from build123d import *

# Parameters (mm, degrees)
SKETCH1_R           = 25.4
BOSS_EXTRUDE1_DEPTH = 81.407
SKETCH2_R           = 3.81
CUT_EXTRUDE2_DEPTH  = 167.729477286


with BuildPart() as part:
    # Sketch1 → Boss-Extrude1 (new, symmetric)
    with BuildSketch(Plane.XY):
        Circle(SKETCH1_R)
    extrude(amount=BOSS_EXTRUDE1_DEPTH, both=True)

    # Sketch2 → Cut-Extrude2 (cut, through all)
    with BuildSketch(Plane.XY.offset(81.407)):
        Circle(SKETCH2_R)
    extrude(amount=-CUT_EXTRUDE2_DEPTH, mode=Mode.SUBTRACT)

    # Sketch6 → Cut-Revolve1 (revolve, cut)
    with BuildSketch(Plane(origin=(0, 0, 0), x_dir=(0, 0, -1), z_dir=(1, 0, 0)), mode=Mode.PRIVATE) as cut_revolve1_sk:
        Polygon((-12.207313926, 0), (-81.407, 18.542), (-81.407, 0), align=None)
    revolve(cut_revolve1_sk.sketch.rotate(Axis((0, 0, -89.5477), (0, 0, 1)), 270), axis=Axis((0, 0, -89.5477), (0, 0, 1)), mode=Mode.SUBTRACT)


solid = part.part
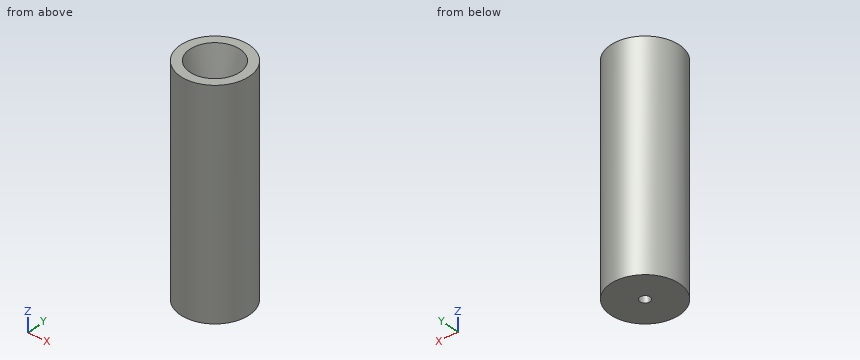
Read the model definition and answer for the solid it produces. Units are mm, in the model's axes. Give positions to 0.01 mm unless a question says otherwise; leave off trailing zeros. Write each loop counter-clockwise with the first axis right and the second up, starting at its lowest first coordinate (ties: lowest second). Pieces come first, ordered by that corner, then holes. Notation, with made-up numbers: (71.5, 52.5) -> (113.5, 52.5) arc R11 ccw to (113.5, 61.5) -> close; hole circle Ø5 at (-8, 0.5). An arc over 180 degrees is marked (long way). Answer as a JSON object with one key per item and string values. Group by question number.
1) Consider L1, parallel to Y at x = 0, z = -32; L2, parallel to Y at x = -3.5, z = -52; L3, parallel to Y at x = -9, z = -16. Determine where each line is inside the solid, lowest interval first. Write a range as from..to.
2) Find section D-D (y = -21.5). Write down the section's boundary in (x, z), and give its area (3 significant figures).
3) Find section C-C (z = -64). Write down the section's boundary in (x, y).
4) Each of these flat-tipped pins is pushed along its axis until it touches: P1, Ø8, axis at x = -10, z = 25.5, coming from the +Y side; P2, Ø2, axis at y = 13, z = 23.5, coming from the -X side; P3, Ø12, axis at y = -12.5, z = -44, coming from the +X side. Where does it stop, or does it pass through?
5) Find section A-A (y = 0). Write down the section's boundary in (x, z), and give its area (3 significant figures).
Values follow:
{
 "1": {"L1": "y = -25.4..-3.81, 3.81..25.4", "L2": "y = -25.16..-1.51, 1.51..25.16", "L3": "y = -23.75..23.75"},
 "2": {"outline": "(-13.52, -81.41) -> (13.52, -81.41) -> (13.52, 81.41) -> (-13.52, 81.41) -> close", "area": "4,400 mm2"},
 "3": {"outline": "circle Ø50.8 at (0, 0); hole circle Ø7.62 at (0, 0)"},
 "4": {"P1": "stops at y = 24.68", "P2": "stops at x = -22.39", "P3": "stops at x = 24.55"},
 "5": {"outline": "(-25.4, -81.41) -> (-3.81, -81.41) -> (-3.81, 26.43) -> (-18.54, 81.41) -> (-25.4, 81.41) -> close; (3.81, -81.41) -> (25.4, -81.41) -> (25.4, 81.41) -> (18.54, 81.41) -> (3.81, 26.43) -> close", "area": "6,220 mm2"}
}
